Here's how the part is built. I have some questions about the finished solid (model axes, mm). A direction names the side the tool comes from. Round coordinates to 2 decimals unless told otherwise and drop trailing zeros. Write each loop counter-clockwise with the first axis right and the second up, starting at its lowest first coordinate (ties: lowest second). Pieces come first, ordered by that corner, then holes. Notation, with made-up numbers: (-21.5, 53.25) -> (19.5, 53.25) arc R22 cw to (19.5, 83.25) -> close; hole circle Ø10 at (65.5, -12.75). An arc over 180 degrees is marked (long way). Answer in a Markdown table with one row per item.
from build123d import *

# Parameters (mm, degrees)
SKETCH1_R           = 12.7
BOSS_EXTRUDE1_DEPTH = 2.032
SKETCH2_R           = 12.7
SKETCH2_R_2         = 3.429
BOSS_EXTRUDE2_DEPTH = 2.54
FILLET1_R           = 2.54
FILLET2_R           = 0.635


with BuildPart() as part:
    # Sketch1 → Boss-Extrude1 (new body)
    with BuildSketch(Plane(origin=(0, 0, 0), x_dir=(1, 0, 0), z_dir=(0, 1, 0))):
        with Locations(Location((0, 0, 0), (0, 0, 270))):
            Circle(SKETCH1_R)
        Polygon((7.478995387, 0), (3.739497694, 6.477), (-3.739497694, 6.477), (-7.478995387, 0), (-3.739497694, -6.477), (3.739497694, -6.477), align=None, mode=Mode.SUBTRACT)
    extrude(amount=BOSS_EXTRUDE1_DEPTH)

    # Sketch2 → Boss-Extrude2 (add)
    with BuildSketch(Plane(origin=(0, 2.032, 0), x_dir=(1, 0, 0), z_dir=(0, 1, 0))):
        with Locations(Location((0, 0, 0), (0, 0, 270))):
            Circle(SKETCH2_R)
        with Locations(Location((0, 0, 0), (0, 0, 270))):
            Circle(SKETCH2_R_2, mode=Mode.SUBTRACT)
    extrude(amount=BOSS_EXTRUDE2_DEPTH)

    # Fillet1
    fillet1_edges = [part.edges().sort_by_distance(p)[0] for p in [
        (0, 4.572, -12.7),
    ]]
    fillet(fillet1_edges, radius=FILLET1_R)

    # Fillet2
    fillet2_edges = [part.edges().sort_by_distance(p)[0] for p in [
        (0, 0, -6.477),
        (-5.60924654, 0, -3.2385),
        (-5.60924654, 0, 3.2385),
        (0, 0, 6.477),
        (0, 0, -12.7),
        (5.60924654, 0, 3.2385),
        (5.60924654, 0, -3.2385),
    ]]
    fillet(fillet2_edges, radius=FILLET2_R)


solid = part.part
1) I need wall thicknesses on line 1 (X direction, y = 2.25, z = 0.75); line 2 (Z direction, x = -1, y = 3.4); line 3 (X direction, y = 4.05, z = -0.5). Which ranges of each line are inside material? Lowest first, please. Write a range as [from, to].
Response:
| item | result |
|---|---|
| line 1 | x = [-12.67, -3.35], [3.35, 12.67] |
| line 2 | z = [-12.26, -3.28], [3.28, 12.26] |
| line 3 | x = [-11.69, -3.39], [3.39, 11.69] |
2) We'd pull the mould along Z, two halves only. Please class faces 1 (the face through (-7.7, 1.3, -10.1)), 2 (the face through (0, 4.572, 4)), 3 (the face through (-3.35, 3.28, -0.74)): +Z half, -Z half, draft (parallel to the pull), parting line (faces both ways), or undercut.
Response:
| item | result |
|---|---|
| face 1 | parting line |
| face 2 | draft |
| face 3 | undercut |
3) I want a section at B-B, the plane y = 1.35. List the corners of the cut face in (x, z) for me, and give its area (3 significant figures).
Response:
| item | result |
|---|---|
| outline | circle Ø25.4 at (0, 0); hole (-7.48, 0) -> (-3.74, -6.48) -> (3.74, -6.48) -> (7.48, 0) -> (3.74, 6.48) -> (-3.74, 6.48) -> close |
| area | 361 mm^2 |
4) For pin 1 (6 mm diameter, centred on x = 0, z = 0, fed in from -Y); pin 2 (1.5 mm diameter, centred on x = -1.5, y = 1.5, fed in from -Z); pin 3 (2 mm diameter, centred on x = 5, y = 3.5, fed in from -Z); pin 4 (6.5 mm diameter, centred on x = 1, z = -2.5, fed in from -Y), each with a flat end and sliding along its axis, tell me the tip position at first contact or that it passes through.
Response:
| item | result |
|---|---|
| pin 1 | passes through |
| pin 2 | stops at z = -12.68 |
| pin 3 | stops at z = -11.83 |
| pin 4 | stops at y = 2.03 |
5) I want a section at C-C, the plane y = 3.45. List the corners of the cut face in (x, z) for me, and give its area (3 significant figures).
Response:
| item | result |
|---|---|
| outline | circle Ø24.53 at (0, 0); hole circle Ø6.86 at (0, 0) |
| area | 436 mm^2 |
6) Which directions (+Z, -Z, +X, -X, +Y, -Y) give clear straight access to the entire face, cutting with the end or side of a thin tool? Please do faces 4 (the face through (5.635, 1.324, -3.193)), 5 (the face through (6, 0, 5)).
Response:
| item | result |
|---|---|
| face 4 | -Y |
| face 5 | +Z, -Z, +X, -X, -Y |
7) I want a section at A-A, the plane x = 0. List the corners of the cut face in (y, z) for me (3 decimals).
Response:
| item | result |
|---|---|
| outline | (0, -12.065) arc R0.635 ccw to (0.635, -12.7) -> (2.032, -12.7) arc R2.54 ccw to (4.572, -10.16) -> (4.572, -3.429) -> (2.032, -3.429) -> (2.032, -6.477) -> (0.635, -6.477) arc R0.635 ccw to (0, -7.112) -> close; (0, 7.112) arc R0.635 ccw to (0.635, 6.477) -> (2.032, 6.477) -> (2.032, 3.429) -> (4.572, 3.429) -> (4.572, 10.16) arc R2.54 ccw to (2.032, 12.7) -> (0.635, 12.7) arc R0.635 ccw to (0, 12.065) -> close |
